from build123d import *

# Parameters (mm, degrees)
SKETCH1_W           = 125
SKETCH1_H           = 115
BOSS_EXTRUDE1_DEPTH = 6.88
SKETCH2_W           = 10
SKETCH2_H           = 13.6
SKETCH2_W_2         = 12
BOSS_EXTRUDE2_DEPTH = 6.88
SKETCH3_W           = 13.76
SKETCH3_H           = 89
BOSS_EXTRUDE3_DEPTH = 6.88
FILLET1_R           = 2.5


with BuildPart() as part:
    # Sketch1 → Boss-Extrude1 (new body)
    with BuildSketch(Plane.XY):
        Rectangle(SKETCH1_W, SKETCH1_H)
    extrude(amount=BOSS_EXTRUDE1_DEPTH)

    # Sketch2 → Boss-Extrude2 (add)
    with BuildSketch(Plane.XY.offset(6.88)):
        with Locations((-52.5, 57.5)):
            Rectangle(SKETCH2_W, SKETCH2_H)
        with Locations((-22.5, 57.5)):
            Rectangle(SKETCH2_W, SKETCH2_H)
        with Locations((-41.5, -57.5)):
            Rectangle(SKETCH2_W_2, SKETCH2_H)
        with Locations((41.5, -57.5)):
            Rectangle(SKETCH2_W_2, SKETCH2_H)
    extrude(amount=-BOSS_EXTRUDE2_DEPTH)

    # Sketch3 → Boss-Extrude3 (add)
    with BuildSketch(Plane.XY.offset(6.88)):
        with Locations((62.5, 0)):
            Rectangle(SKETCH3_W, SKETCH3_H)
    extrude(amount=-BOSS_EXTRUDE3_DEPTH)

    # Fillet1
    fillet1_edges = [part.edges().sort_by_distance(p)[0] for p in [
        (69.38, -44.5, 3.44),
        (69.38, 44.5, 3.44),
        (-47.5, 64.3, 3.44),
        (-57.5, 64.3, 3.44),
        (-17.5, 64.3, 3.44),
        (-27.5, 64.3, 3.44),
        (-47.5, -64.3, 3.44),
        (-35.5, -64.3, 3.44),
        (-62.5, 57.5, 3.44),
        (62.5, 57.5, 3.44),
        (35.5, -64.3, 3.44),
        (62.5, -57.5, 3.44),
        (-62.5, -57.5, 3.44),
        (47.5, -64.3, 3.44),
    ]]
    fillet(fillet1_edges, radius=FILLET1_R)


solid = part.part
Geometry: final body of the model. Coordinates: model frame, mm. A direction names the side the tool comes from. Coordinates: 2 decimals unless noted, no trailing zeros. Loops run counter-clockwise (first coordinate to the right, second up) from the corner with the lowest first, then second, coordinate; pieces in that order, holes last. Notation, with made-up numbers: (-11.75, 58.25) - (6.25, 58.25) arc R10 ccw to (6.25, 75.25) - close; hole circle Ø10 at (35.25, -6). An arc over 180 degrees is marked (long way). Put each result on its own line as item: value. Start each with the question number.
Q1. Pull-direction query (X, two-part tool) for faces 4 (the flat face through (-47.5, -60, 3)), 5 (the flat face through (0, -57.5, 3)), 6 (the flat face through (35.5, -60, 3)), 7 (the flat face through (47.5, -60, 3)); classes: released by +X, released by -X, zero draft, split by the parting line, or undercut.
Q2. Cut plane B-B, the plane y = 50. Return loops of the section in (x, z).
Q3. Pin query (flat end, axial travel): pin 1 Ø2 at (x, z) = (-59, 2.5) entering from +Y; pin 2 Ø1.3 at (y, z) = (58.5, 3.5) entering from -X; pin 3 Ø3.5 at (y, z) = (60, 3) entering from +X. Return the tip coordinate at first contact, or that it passes through.
Q4. Set-up query: faces 1 (the flat face through (-17.5, 60, 3)), 2 (the flat face through (-35.5, -60, 3)), 3 (the flat face through (-38, 57.5, 3)). Return all of +Z, -Z, +X, -X, +Y, -Y with unobstructed straight access to the full face (end or side cutting, diameter ignored); none if empty.
Q5. Line query: line 1 (X direction, y = 53, z = 3.5); line 2 (Y direction, x = 22, z = 3.5); line 3 (Y direction, x = -20, z = 2.5). Output: solid intervals per line, ascending.
Q6. Cut plane A-A, the plane x = 32. Return loops of the section in (y, z).
Filled sheet:
1. face 4: released by -X
1. face 5: undercut
1. face 6: undercut
1. face 7: released by +X
2. outline: (-62.5, 0) - (62.5, 0) - (62.5, 6.88) - (-62.5, 6.88) - close
3. pin 1: y = 57.5
3. pin 2: x = -57.5
3. pin 3: x = -17.5
4. face 1: +Z, -Z, +X, +Y
4. face 2: +Z, -Z, -Y
4. face 3: +Z, -Z, +Y
5. line 1: -62.5 to 62.5
5. line 2: -57.5 to 57.5
5. line 3: -57.5 to 64.3
6. outline: (-57.5, 0) - (57.5, 0) - (57.5, 6.88) - (-57.5, 6.88) - close
